Input: part model. Units: mm. Frame: model coordinates. Give positions to 0.01 mm unless a question says otherwise; leave off trailing zeros. Loops run counter-clockwise (first coordinate to the right, second up) from the corner with the lowest first, then second, coordinate; pieces in that order, holes last. Notation, with made-up numbers: M -14.75,-4 L 42.25,-4 A16 ccw 42.25,26 Z; hole C -35,9 d5. An arc over 180 degrees is marked long. Use a Markdown table: item, result. Add a question column.
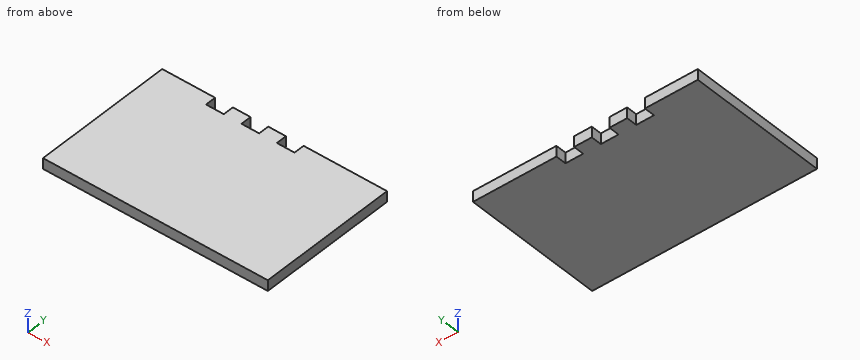
Autodesk Inventor part; units mm, degrees
ref_plane "YZ Plane" through (0, 0, 0) normal (1, 0, 0) x (0, 1, 0)
ref_plane "XZ Plane" through (0, 0, 0) normal (0, 1, 0) x (-1, 0, 0)
ref_plane "XY Plane" through (0, 0, 0) normal (0, 0, 1) x (1, 0, 0)
sketch "Sketch1" plane through (0, 0, 0) normal (0, 0, 1) x (1, 0, 0)
  line L0 (0, -129) -> (0, 146.2673)
  line L1 (-130, -1) -> (-130, 5)
  line L2 (-10, 5) -> (0, 5)
  line L3 (0, -74) -> (-450, -74)
  line L4 (-130, 5) -> (-120, 5)
  line L5 (0, -74) -> (-129.8, -74)
  line L6 (-129.8, -68) -> (-129.8, -74)
  line L7 (0, 5) -> (-129.9001, 5)
  line L8 (-129.9001, 5) -> (-129.9001, -74)
  line L9 (-129.9001, -74) -> (0, -74)
  line L10 (0, -74) -> (0, 5)
  line L11 (-155.5538, 0) -> (-155.5538, 5)
  line L12 (-170.1, 0) -> (-170.1, 5)
  point P0 (0, 0)
  point P1 (-129.9001, -74)
  point P2 (-120, 5)
  point P3 (-130, 0)
  point P4 (-129.9001, 5)
  point P5 (-129.9001, 5)
extrude "Extrusion1" add sketch "Sketch1" along normal blind 6
ref_plane "Work Plane2" through (-20.1, 0, 6) normal (0, 1, 0) x (1, 0, 0)
sketch "Sketch3" plane through (-20.1, 0, 6) normal (0, 1, 0) x (1, 0, 0)
  circle A0 centre (5.1, 3) radius 1.5
  point P0 (20.1, 6)
hole "Hole1" at (-15, 0, 3) direction (0, -1, 0) diameter 2.8 depth 20
ref_plane "Work Plane1" through (-129.9001, -34.5, 0) normal (0, -1, 0) x (1, 0, 0)
sketch "Skizze4" plane through (0, 0, 6) normal (0, 0, 1) x (1, 0, 0)
  line L0 (-2.3877, -54.9) -> (-2.3877, -60)
  line L1 (16.4895, -81.7963) -> (-2.8877, -81.7963)
  line L2 (-2.8877, -81.7963) -> (-2.8877, 13.3495)
  line L3 (-2.8877, 13.3495) -> (16.4895, 13.3495)
  line L4 (16.4895, 13.3495) -> (16.4895, -81.7963)
  point P0 (0, 0)
  dimension "d23" = 0.5
extrude "Extrusion3" cut sketch "Skizze4" against normal blind 10
sketch "Sketch6" plane through (0, 0, 6) normal (0, 0, 1) x (1, 0, 0)
  line L0 (-100, 5) -> (-100, -1)
  line L1 (-100, -1) -> (-90, -1)
  line L2 (-90, -1) -> (-90, 5)
  line L3 (-2.8877, 5) -> (-129.9001, 5)
  point P0 (0, 0)
  point P1 (-100, 5)
  point P2 (-90, 5)
extrude "Extrusion5" cut sketch "Sketch6" against normal through all
pattern_linear "Rectangular Pattern3" count 3 spacing 20 along (1, 0, 0) of "Extrusion5"
properties part number "00_Baseplate_Simmo_side6"
1) Ray query, line 1 (X direction, y = -15.5, z = 3); line 2 (Z direction, x = -15, y = -12.25); line 3 (Y direction, x = -52.5, z = 2.5). Return the intervals inside material, ascending. Write a range as [from, to].
2) Contact query for a flat-ended pin moving along its axis: P1, Ø1.8, axis at x = -72.5, z = 4, coming from the +Y side. Output: stop coordinate, or through.
3) Section query A-A, the plane z = 3. Return the cut outline in (x, y).
4) Section query B-B, the plane x = -15. Return the cut outline in (y, z).
5) Section query C-C, the plane x = -76. Return the cut outline in (y, z), and give its area (3 significant figures).
Entries:
| question | item | result |
|---|---|---|
| 1 | line 1 | x = [-129.9, -16.4], [-13.6, -2.89] |
| 1 | line 2 | z = [0, 1.6], [4.4, 6] |
| 1 | line 3 | y = [-74, -1] |
| 2 | P1 | stops at y = -1 |
| 3 | outline | M -129.9,-74 L -2.89,-74 L -2.89,5 L -50,5 L -50,-1 L -60,-1 L -60,5 L -70,5 L -70,-1 L -80,-1 L -80,5 L -90,5 L -90,-1 L -100,-1 L -100,5 L -129.9,5 Z; hole M -16.4,-20 L -13.6,-20 L -13.6,0 L -16.4,0 Z |
| 4 | outline | M -74,0 L 5,0 L 5,6 L -74,6 Z; hole M -20,1.6 L 0,1.6 L 0,4.4 L -20,4.4 Z |
| 5 | outline | M -74,0 L -1,0 L -1,6 L -74,6 Z |
| 5 | area | 438 mm² |
